The listing builds one solid part. Answer for the finished solid, in the listing's coordinates (mm). A direction names the side the tool comes from. Coordinates: 2 decimals unless noted, no trailing zeros. Loops run counter-clockwise (first coordinate to the right, second up) from the corner with the lowest first, then second, coordinate; pieces in that order, holes last. Notation, with made-up numbers: M 70,-10 L 104,-10 A10 ccw 104,4 Z; hole C -4,-8.75 d6. An arc over 180 degrees is marked long. Return JSON: item names as keys, results as strings. Group by question number.
1. Section D-D (z = 14.5) is taken. Write down the section's boundary in (x, y).
2. Section C-C (z = 1.5) is taken. Write down the section's boundary in (x, y).
3. The mould has two halves that part along Y. Classify faces 1 (the face through (-1.08, -4.88, 10.92)), 2 (the face through (0, 10, 2)), 3 (the face through (0, -10, 2)), 4 (the face through (0, 0, 5)): pulls with the +Y half, pulls with the -Y half, needs draft (parallel to the pull), parting line crosses it, or undercut.
4. Straight lines are drawn through the part: L1, parallel to Y at x = 0, z = 13.25; L2, parallel to Z at x = -2.25, y = -1; L3, parallel to Y at x = -4, z = 10.5. For each, find the intervals that lie inside material, in ascending order. Write a range as from..to.
5. Which of the six approach directions +Z, -Z, +X, -X, +Y, -Y give full straight-line access (tool end or side, diameter ignored) to faces 5 (the face through (-9, 0, 5)), 6 (the face through (-11.289, 8.196, 2.535))?
6. Section B-B (y = 0) is taken. Write down the section's boundary in (x, z), then the cut area to 3 significant figures.
7. Given P1, Ø6, axis at y = 2, z = 14.5, coming from the -X side; P2, Ø1.5, axis at y = 5, z = 3.5, coming from the +X side; P3, Ø1, axis at x = -9.5, y = 7.5, coming from the -Z side; P4, Ø8, axis at y = 3, z = 14, coming from the +X side, each flat-ended and moving along its own axis, determine where each tip first touches the part or whether it passes through.
8. Section A-A (x = 0) is taken. Write down the section's boundary in (y, z).
```python
from build123d import *

# Parameters (mm, degrees)
SKETCH_1_W      = 26
SKETCH_1_H      = 20
EXTRUDE_1_DEPTH = 5
SKETCH_2_R      = 8
SKETCH_2_R_2    = 5
EXTRUDE_2_DEPTH = 12
FILLET_1_R      = 6


with BuildPart() as part:
    # 草图1 → 凸台-拉伸1 (new body)
    with BuildSketch(Plane.XY):
        Rectangle(SKETCH_1_W, SKETCH_1_H)
    extrude(amount=EXTRUDE_1_DEPTH)

    # 草图2 → 凸台-拉伸2 (add)
    with BuildSketch(Plane.XY.offset(5)):
        Circle(SKETCH_2_R)
        Circle(SKETCH_2_R_2, mode=Mode.SUBTRACT)
    extrude(amount=EXTRUDE_2_DEPTH)

    # 圆角1
    fillet_1_edges = [part.edges().sort_by_distance(p)[0] for p in [
        (13, 10, 2.5),
        (13, -10, 2.5),
        (-13, -10, 2.5),
        (-13, 10, 2.5),
    ]]
    fillet(fillet_1_edges, radius=FILLET_1_R)


solid = part.part
```
Worked out:
{
 "1": {"outline": "C 0,0 d16; hole C 0,0 d10"},
 "2": {"outline": "M -13,-4 A6 ccw -7,-10 L 7,-10 A6 ccw 13,-4 L 13,4 A6 ccw 7,10 L -7,10 A6 ccw -13,4 Z"},
 "3": {"face 1": "undercut", "face 2": "pulls with the +Y half", "face 3": "pulls with the -Y half", "face 4": "undercut"},
 "4": {"L1": "-8..-5, 5..8", "L2": "0..5", "L3": "-6.93..-3, 3..6.93"},
 "5": {"face 5": "+Z", "face 6": "+Z, -Z, -X, +Y"},
 "6": {"outline": "M -13,0 L 13,0 L 13,5 L 8,5 L 8,17 L 5,17 L 5,5 L -5,5 L -5,17 L -8,17 L -8,5 L -13,5 Z", "area": "202 mm^2"},
 "7": {"P1": "x = -8", "P2": "x = 12.99", "P3": "z = 0", "P4": "x = 8"},
 "8": {"outline": "M -10,0 L 10,0 L 10,5 L 8,5 L 8,17 L 5,17 L 5,5 L -5,5 L -5,17 L -8,17 L -8,5 L -10,5 Z"}
}
